Verification items for the finished model (mm, model axes). Coordinates: 2 decimals unless noted, no trailing zeros. Order: outer loops, then holes, each group sorted by start corner. A loop starts at its lowest first (then second) coordinate and runs counter-clockwise, first axis right, second up. Notation, with made-up numbers: M -22,42.25 L 15,42.25 A13 cw 15,62.25 Z; hole C 26.5,-19 d8. An arc over 180 degrees is marked long. Use one line per item in the form item = value. Start each with the question number.
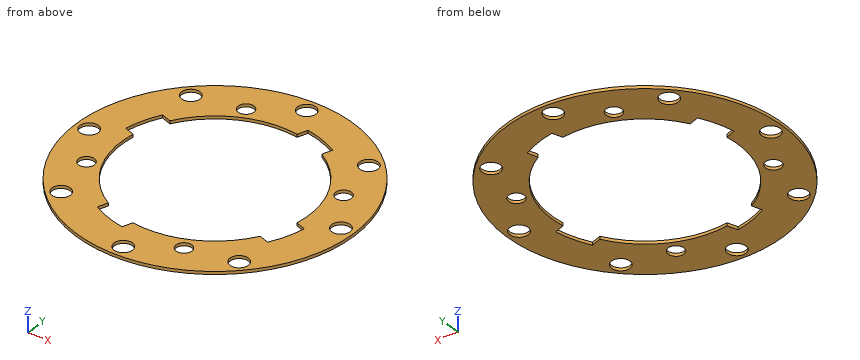
```python
from build123d import *

# Parameters (mm, degrees)
F0_R            = 301.625
F0_R_2          = 17.145
F0_R_3          = 20.0025
F1_DEPTH        = 6.35
F2_DEPTH        = 6.351
F2_COPIES_COUNT = 8
F3_DEPTH        = 6.351
F3_COPIES_COUNT = 4
F4_DEPTH        = 6.351
F4_COPIES_COUNT = 4


# Not quite as in the source:
# - a pattern or mirror of a feature is missing from the dataset's text; its kind, count and spacing are read off the source's solid


with BuildPart() as f1:
    # F0 (on Top) → F1 (new body)
    with BuildSketch(Plane.XY):
        Circle(F0_R)
        with Locations((-88.6964525364, 214.1321786478)):
            Circle(F0_R_2, mode=Mode.SUBTRACT)
        with BuildLine():
            ThreePointArc((104.6230881005, 174.1960086693), (176.846899184, 100.0770415679), (203.2, 0))
            ThreePointArc((203.2, 0), (-154.5268592771, -131.9533620714), (31.8251007682, 200.6923091728))
            Line((31.8251007682, 200.6923091728), (39.7746000853, 222.5333790425))
            ThreePointArc((39.7746000853, 222.5333790425), (77.3170736002, 212.4269138549), (112.5725874176, 196.037078539))
            Line((112.5725874176, 196.037078539), (104.6230881005, 174.1960086693))
        make_face(mode=Mode.SUBTRACT)
        with Locations((0, 273.05)):
            Circle(F0_R_3, mode=Mode.SUBTRACT)
        with BuildLine():
            ThreePointArc((31.8251007682, 200.6923091728), (69.4984931238, 190.9455405437), (104.6230881005, 174.1960086693))
            Line((104.6230881005, 174.1960086693), (112.5725874176, 196.037078539))
            ThreePointArc((112.5725874176, 196.037078539), (77.3170736002, 212.4269138549), (39.7746000853, 222.5333790425))
            Line((39.7746000853, 222.5333790425), (31.8251007682, 200.6923091728))
        make_face()
        with Locations((0, 273.05)):
            Circle(F0_R_3)
        with Locations((-88.6964525364, 214.1321786478)):
            Circle(F0_R_2)
    extrude(amount=F1_DEPTH)

    # F0 (on Top) → F2 (cut, through all)
    with BuildSketch(Plane.XY):
        with Locations((0, 273.05)):
            Circle(F0_R_3)
    f2 = extrude(amount=F2_DEPTH, mode=Mode.SUBTRACT)

    # F2_copies: F2 ×8 about axis
    f2_copies_axis = Axis((0, 0, 0), (0, 0, 1))
    for i in range(1, F2_COPIES_COUNT):
        add(f2.rotate(f2_copies_axis, i * 360 / F2_COPIES_COUNT), mode=Mode.SUBTRACT)

    # F0 (on Top) → F3 (cut, through all)
    with BuildSketch(Plane.XY):
        with BuildLine():
            ThreePointArc((31.8251007682, 200.6923091728), (69.4984931238, 190.9455405437), (104.6230881005, 174.1960086693))
            Line((104.6230881005, 174.1960086693), (112.5725874176, 196.037078539))
            ThreePointArc((112.5725874176, 196.037078539), (77.3170736002, 212.4269138549), (39.7746000853, 222.5333790425))
            Line((39.7746000853, 222.5333790425), (31.8251007682, 200.6923091728))
        make_face()
    f3 = extrude(amount=F3_DEPTH, mode=Mode.SUBTRACT)

    # F3_copies: F3 ×4 about axis
    f3_copies_axis = Axis((0, 0, 0), (0, 0, 1))
    for i in range(1, F3_COPIES_COUNT):
        add(f3.rotate(f3_copies_axis, i * 360 / F3_COPIES_COUNT), mode=Mode.SUBTRACT)

    # F0 (on Top) → F4 (cut, through all)
    with BuildSketch(Plane.XY):
        with Locations((-88.6964525364, 214.1321786478)):
            Circle(F0_R_2)
    f4 = extrude(amount=F4_DEPTH, mode=Mode.SUBTRACT)

    # F4_copies: F4 ×4 about axis
    f4_copies_axis = Axis((0, 0, 0), (0, 0, 1))
    for i in range(1, F4_COPIES_COUNT):
        add(f4.rotate(f4_copies_axis, i * 360 / F4_COPIES_COUNT), mode=Mode.SUBTRACT)


solid = f1.part
```
1. Depth check by flat-ended pin: P1, Ø1, axis at y = 221.5, z = 5, coming from the +X side; P2, Ø20.5, axis at x = 88.7, y = -214.13, coming from the +Z side. Enter the tip coordinate at first touch or a pass-through.
2. Cross-section at A-A on y = 0. Give the number of separate pieces and of enclosed holes in the cut face, and give its area (3 significant figures).
3. Cross-section at D-D on y = -62. Enter the section's corners in (x, z).
4. Material ranges on line 1 along Y through (x, z) = (0, 3.75) (1 decimal); line 2 along X through (y, z) = (83, 0.5); line 3 along Y through (x, z) = (81, 5.5), recorded low to high.
Final values:
q1.P1 = 205.27
q1.P2 = through
q2.separate_pieces = 4
q2.enclosed_holes = 0
q2.area = 742 mm2
q3.outline = M -295.18,0 L -193.51,0 L -193.51,6.35 L -295.18,6.35 Z; M 217.39,0 L 295.18,0 L 295.18,6.35 L 217.39,6.35 Z
q4.line_1 = -301.6 to -293.1, -253 to -203.2, 203.2 to 253, 293.1 to 301.6
q4.line_2 = -289.98 to -210.27, 185.48 to 197.96, 230.3 to 289.98
q4.line_3 = -290.55 to -229.45, -198.81 to -186.36, 211.05 to 290.55
